Source: CAD feature listing. Evaluate the final solid. Frame: model axes, mm. Face numbers are marked on the shaded views. A direction names the side the tool comes from. Give positions to 0.01 mm unless a question says otherwise; leave off trailing zeros. Order: outer loops, then holes, each group sorted by start corner. A loop starts at its lowest first (then second) coordinate and runs counter-clockwise, first axis right, second up.
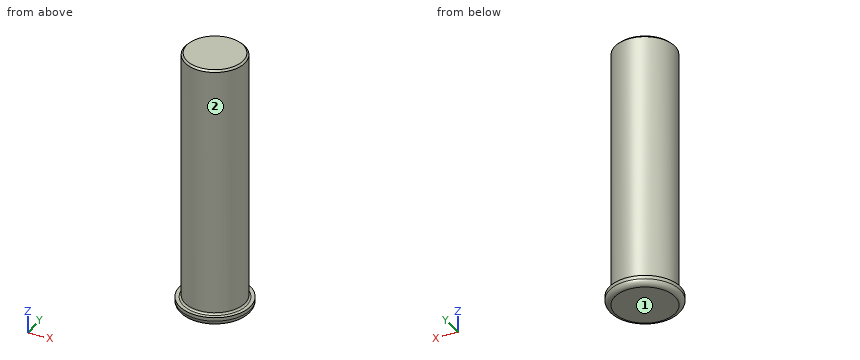
from build123d import *

# Parameters (mm, degrees)
SCHIZZO1_R                   = 10
ESTRUSIONE_ESTRUSIONE1_DEPTH = 2.5
SCHIZZO2_R                   = 8.45
ESTRUSIONE_ESTRUSIONE2_DEPTH = 71.5
RACCORDO1_R                  = 0.5
SMUSSO2_SIZE                 = 0.5
RACCORDO3_R                  = 1.5


with BuildPart() as part:
    # Schizzo1 → Estrusione-Estrusione1 (new body)
    with BuildSketch(Plane.XY):
        with Locations((0, 2.505612013)):
            Circle(SCHIZZO1_R)
    extrude(amount=ESTRUSIONE_ESTRUSIONE1_DEPTH)

    # Schizzo2 → Estrusione-Estrusione2 (add)
    with BuildSketch(Plane.XY.offset(2.5)):
        with Locations((0, 2.505612013)):
            Circle(SCHIZZO2_R)
    extrude(amount=ESTRUSIONE_ESTRUSIONE2_DEPTH)

    # Raccordo1
    raccordo1_edges = [part.edges().sort_by_distance(p)[0] for p in [
        (-8.45, 2.505612013, 2.5),
    ]]
    fillet(raccordo1_edges, radius=RACCORDO1_R)

    # Smusso2
    smusso2_edges = [part.edges().sort_by_distance(p)[0] for p in [
        (-8.45, 2.505612013, 74),
    ]]
    chamfer(smusso2_edges, length=SMUSSO2_SIZE)

    # Raccordo3
    raccordo3_edges = [part.edges().sort_by_distance(p)[0] for p in [
        (-10, 2.505612013, 0),
    ]]
    fillet(raccordo3_edges, radius=RACCORDO3_R)


solid = part.part
1) Ray query, L1, parallel to X at y = 3, z = 63; L2, parallel to Y at x = 7.75, z = 23; L3, parallel to X at y = 10, z = 46. Return the intervals inside material, ascending.
Checks:
L1: x = -8.44 to 8.44
L2: y = -0.86 to 5.87
L3: x = -3.9 to 3.9
2) First-contact query: pin 1 Ø4 at (y, z) = (3.5, 12.5) entering from -X; pin 2 Ø12 at (x, z) = (6.5, 36) entering from +Y; pin 3 Ø2 at (y, z) = (-5.5, 10.5) entering from +X; pin 4 Ø6 at (x, y) = (-7, -5) entering from -Z. Flat tips, straight axial feed; report the tip coordinate or a pass-through.
Checks:
pin 1: stops at x = -8.45
pin 2: stops at y = 10.94
pin 3: stops at x = 4.72
pin 4: stops at z = 0
3) Reachability of the marked faces 1 and 2 from +Z, -Z, +X, -X, +Y, -Y: full face, straight path, thin tool, end or side. Return the list, or none.
Checks:
face 1: -Z, +X, -X, +Y, -Y
face 2: +Z
4) Section query B-B on z = 62. Output: boundary loops of the cut face in (x, y), and give its area (3 significant figures).
Checks:
outline: circle Ø16.9 at (0, 2.51)
area: 224 mm2
5) Section query A-A on x = 0. Output: boundary loops of the cut face in (y, z).
Checks:
outline: (-7.49, 1.5) arc R1.5 ccw to (-5.99, 0) - (11.01, 0) arc R1.5 ccw to (12.51, 1.5) - (12.51, 2.5) - (11.46, 2.5) arc R0.5 cw to (10.96, 3) - (10.96, 73.5) - (10.46, 74) - (-5.44, 74) - (-5.94, 73.5) - (-5.94, 3) arc R0.5 cw to (-6.44, 2.5) - (-7.49, 2.5) - close
